from build123d import *

# Parameters (mm, degrees)
ESBO_O1_W                = 96
ESBO_O1_H                = 136
RESSALTO_EXTRUS_O1_DEPTH = 3
CORTE_EXTRUS_O1_DEPTH    = 10
FILETE1_R                = 8


with BuildPart() as part:
    # Esboço1 → Ressalto-extrusão1 (new body)
    with BuildSketch(Plane.XY):
        Rectangle(ESBO_O1_W, ESBO_O1_H)
    extrude(amount=RESSALTO_EXTRUS_O1_DEPTH)

    # Esboço2 → Corte-extrusão1 (cut)
    with BuildSketch(Plane.XY.offset(3)):
        Polygon((-38, -48.876349567), (-5.977564077, 0), (-38, 48.876349567), align=None)
        Polygon((0, 9.123650433), (32.022435923, 58), (-32.022435923, 58), align=None)
        Polygon((38, -48.876349567), (38, 48.876349567), (5.977564077, 0), align=None)
        Polygon((32.022435923, -58), (0, -9.123650433), (-32.022435923, -58), align=None)
    extrude(amount=-CORTE_EXTRUS_O1_DEPTH, mode=Mode.SUBTRACT)

    # Filete1
    filete1_edges = [part.edges().sort_by_distance(p)[0] for p in [
        (38, 48.876349567, 1.5),
        (38, -48.876349567, 1.5),
        (5.977564077, 0, 1.5),
        (-32.022435923, 58, 1.5),
        (32.022435923, 58, 1.5),
        (0, 9.123650433, 1.5),
        (0, -9.123650433, 1.5),
        (32.022435923, -58, 1.5),
        (-32.022435923, -58, 1.5),
        (-38, 48.876349567, 1.5),
        (-5.977564077, 0, 1.5),
        (-38, -48.876349567, 1.5),
    ]]
    fillet(filete1_edges, radius=FILETE1_R)


solid = part.part
Geometry check sheet. Reference: the model listing, model coordinates, mm. A direction names the side the tool comes from. Coordinates: 2 decimals unless noted, no trailing zeros. Order: outer loops, then holes, each group sorted by start corner. A loop starts at its lowest first (then second) coordinate and runs counter-clockwise, first axis right, second up. Notation, with made-up numbers: (76.5, 57) - (87.5, 57) arc R18 ccw to (87.5, 91) - close; hole circle Ø11 at (-7, 20). An arc over 180 degrees is marked (long way). One line per item, written item: value.
(1) Sectioned sample at B-B (y = -39.5). Enter the section's corners in (x, z), and give its area (3 significant figures).
Data:
outline: (-48, 0) - (-19.9, 0) - (-19.9, 3) - (-48, 3) - close; (19.9, 0) - (48, 0) - (48, 3) - (19.9, 3) - close
area: 169 mm^2
(2) Sectioned sample at D-D (y = 12.5). Enter the section's corners in (x, z).
Data:
outline: (-48, 0) - (-38, 0) - (-38, 3) - (-48, 3) - close; (-14.17, 0) - (14.17, 0) - (14.17, 3) - (-14.17, 3) - close; (38, 0) - (48, 0) - (48, 3) - (38, 3) - close
(3) Sectioned sample at A-A (z = 1.4). Enter the section's corners in (x, y).
Data:
outline: (-48, -68) - (48, -68) - (48, 68) - (-48, 68) - close; hole (-38, -22.07) arc R8 ccw to (-23.31, -26.45) - (-8.85, -4.38) arc R8 ccw to (-8.85, 4.38) - (-23.31, 26.45) arc R8 ccw to (-38, 22.07) - close; hole (-23.91, -45.62) arc R8 ccw to (-17.22, -58) - (17.22, -58) arc R8 ccw to (23.91, -45.62) - (6.69, -19.34) arc R8 ccw to (-6.69, -19.34) - close; hole (-23.91, 45.62) - (-6.69, 19.34) arc R8 ccw to (6.69, 19.34) - (23.91, 45.62) arc R8 ccw to (17.22, 58) - (-17.22, 58) arc R8 ccw to start; hole (8.85, -4.38) - (23.31, -26.45) arc R8 ccw to (38, -22.07) - (38, 22.07) arc R8 ccw to (23.31, 26.45) - (8.85, 4.38) arc R8 ccw to start
(4) Access from +Z, -Z, +X, -X, +Y, -Y to the whole of each face (thin tool, end or side, straight path). Record for faces 1 (the face through (0, 58, 2)), 2 (the face through (-1, 1, 0)).
Data:
face 1: +Z, -Z
face 2: -Z, +X, -X, +Y, -Y
(5) Sectioned sample at C-C (x = 11). Enter the section's corners in (y, z), and give its area (3 significant figures).
Data:
outline: (-68, 0) - (-58, 0) - (-58, 3) - (-68, 3) - close; (-25.91, 0) - (-7.67, 0) - (-7.67, 3) - (-25.91, 3) - close; (7.67, 0) - (25.91, 0) - (25.91, 3) - (7.67, 3) - close; (58, 0) - (68, 0) - (68, 3) - (58, 3) - close
area: 169 mm^2
(6) Thickness scan on probe 1 along Y at (x, z) = (0, 1.75); probe 2 along X at (y, z) = (-9, 0.25); probe 3 along X at (y, z) = (-13, 1.4). Record the ranges inside material, lowest first. Write a range as from..to.
Data:
probe 1: y = -68..-58, -15.72..15.72, 58..68
probe 2: x = -48..-38, -11.87..11.87, 38..48
probe 3: x = -48..-38, -14.49..14.49, 38..48
